Model file for the job. Use its own axes, mm. A direction names the side the tool comes from. Give positions to 0.01 mm unless a question says otherwise; leave off trailing zeros. Loops run counter-clockwise (first coordinate to the right, second up) from the corner with the lowest first, then second, coordinate; pieces in that order, holes last. Notation, with made-up numbers: (-28, 25.5) - (10, 25.5) arc R14 ccw to (10, 40.5) - close; hole circle Ø6 at (73.5, -14.75). An arc over 180 degrees is marked (long way). Answer as CSV lines item,"result". Start each with the question number.
Item 1: Saw through at B-B on z = 0. Give the cut face in (x, y) (3 decimals), plus the area to 3 significant figures.
Item 2: Drill centre lines: L1, parallel to X at y = -0.1, z = 1.5; L2, parallel to Z at x = 10.5, y = -0.2; L3, parallel to X at y = -0.9, z = 7.5. Where is each one in solid material? Low to high. Write a range as from..to.
Item 3: Saw through at D-D on z = -11.5. Give the cut face in (x, y), plus the area to 3 significant figures.
Item 4: Pin check, flat tip, straight feed: pin 1 (0.6 mm diameter, centred on y = -1, z = -7, fed in from +X). Stop position of the tip, or through.
Item 5: Pull direction Z, two halves, no side cores. Call faces 3 (the flat face through (6.747, -0.986, -3.44)), 4 (the cylindrical face through (-0.519, -0.986, -17.993)), 5 (the flat face through (0, 0, 1)): pulls with the +Z half, pulls with the -Z half, needs draft (parallel to the pull), parting line crosses it, or undercut.
Item 6: Tool access for faces 1 (the flat face through (-6.65, -0.99, -3.67)), 2 (the flat face through (0, -2, 1)): list every direction of +Z, -Z, +X, -X, +Y, -Y with a clear straight run to the whole face (end or side of a thin tool).
Item 7: Saw through at C-C on y = -0.5. State how many separate pieces and enclosed holes the cut face has, plus the area to 3 significant figures.
Item 8: Saw through at A-A on z = 16.5. Give the cut face in (x, y), plus the area to 3 significant figures.
from build123d import *

# Parameters (mm, degrees)
F1_R     = 18
F1_R_2   = 15.375
F2_DEPTH = 2
F3_DEPTH = 2


with BuildPart() as f2:
    # F0 (on Front) + F1 (on Front) → F2 (new body)
    with BuildSketch(Plane.XZ):
        Polygon((-19.759701, 18.612917), (-19.777608, 18.638063), (-19.78312, 18.635015), (-19.838238, 18.599201), (-19.84375, 18.595391), (-19.339382, 17.290085), (-14.268196, 4.150538), (-13.75283, 2.817952), (-13.962278, 2.907538), (-15.865373, 3.71508), (-16.047263, 3.792271), (-16.052775, 3.786734), (-16.102355, 3.723335), (-16.106496, 3.716452), (-15.529103, 2.9861), (-9.7441, -4.321632), (-9.165336, -5.053381), (-7.495159, -7.521448), (-7.584719, -7.543521), (-8.051876, -7.553147), (-8.541055, -7.579309), (-8.64169, -7.611034), (-8.356422, -8.069885), (-5.541086, -12.599518), (-5.259984, -13.050114), (-5.24068, -13.105257), (-5.03809, -13.466293), (-4.838268, -13.77635), (-4.819015, -13.806678), (-4.638472, -14.096086), (-2.836012, -17.000982), (-2.655468, -17.291736), (-1.86309, -17.366158), (-2.00091, -16.493846), (-3.376193, -7.774991), (-3.513988, -6.901307), (-3.62839, -6.829654), (-4.295343, -6.427292), (-4.989855, -6.00837), (-5.116652, -5.929808), (-5.2324, -5.854014), (-6.355512, -5.125034), (-6.465748, -5.053381), (-6.497472, -4.820488), (-6.808902, -2.487473), (-6.840576, -2.240788), (-6.338951, -2.426818), (-1.459332, -4.229303), (-0.975639, -4.408449), (-0.966013, -4.848047), (-0.952221, -9.157183), (-0.928802, -9.578873), (-0.796493, -9.667062), (-0.363779, -9.887534), (0.114376, -9.981235), (0.566395, -9.855835), (0.938454, -9.609176), (1.050087, -9.512706), (1.050087, -4.407078), (1.536522, -4.223791), (6.418834, -2.391004), (6.919214, -2.203577), (6.887464, -2.429612), (6.603492, -4.478757), (6.582918, -4.675784), (6.573266, -4.754347), (6.452108, -5.064404), (6.210808, -5.289017), (6.143244, -5.326228), (6.055106, -5.374462), (5.199355, -5.922924), (5.11114, -5.979439), (5.003648, -6.045581), (4.333951, -6.43829), (3.661435, -6.832422), (3.553943, -6.901307), (3.410661, -7.805293), (1.989887, -16.817696), (1.847952, -17.717541), (2.517673, -17.571466), (2.709215, -17.261408), (4.635703, -14.160856), (4.830013, -13.852169), (4.845202, -13.825957), (5.097348, -13.354685), (5.120792, -13.303707), (5.421198, -12.817246), (8.345424, -8.093304), (8.636254, -7.623404), (8.528558, -7.594498), (8.031226, -7.576566), (7.577836, -7.553147), (7.492492, -7.522845), (9.188704, -5.028565), (9.764776, -4.299585), (15.527782, 2.984729), (16.105124, 3.712337), (16.09979, 3.719195), (16.050006, 3.781222), (16.045688, 3.786734), (15.861284, 3.709568), (13.959586, 2.907538), (13.755624, 2.820746), (14.269466, 4.153306), (19.339306, 17.284751), (19.84375, 18.589549), (19.817588, 18.586755), (19.671538, 18.500141), (19.663156, 18.487695), (18.92046, 17.499635), (11.50112, 7.609383), (10.759694, 6.619977), (10.733532, 6.586906), (10.613644, 6.223102), (10.612374, 6.181776), (10.606786, 6.030189), (10.537952, 4.503318), (10.532364, 4.35036), (8.723122, 1.944319), (8.717534, 1.934642), (8.384032, 2.050415), (8.382508, 2.077974), (8.37438, 2.339797), (8.372856, 2.379777), (8.286242, 2.944749), (7.617714, 4.576343), (6.234176, 6.447739), (4.474489, 7.867193), (3.082671, 8.572551), (2.592095, 8.704885), (2.714727, 9.290609), (3.347263, 12.166651), (3.923284, 14.594637), (4.019728, 14.955825), (3.862629, 15.030247), (2.64447, 15.287803), (1.393957, 15.372972), (0, 13.366205), (-1.320852, 15.286005), (-1.918233, 15.225827), (-3.001366, 15.015007), (-3.598062, 14.824761), (-3.77444, 14.722907), (-3.6449, 14.281963), (-3.07025, 11.840007), (-2.571445, 9.225839), (-2.477694, 8.696757), (-2.965526, 8.557565), (-4.340835, 7.843571), (-6.072988, 6.428435), (-7.433132, 4.572229), (-8.089087, 2.95717), (-8.174533, 2.397658), (-8.177276, 2.365985), (-8.182788, 2.160676), (-8.182788, 2.135835), (-8.239303, 2.116557), (-8.659597, 1.974621), (-8.703691, 1.958061), (-10.526827, 4.382033), (-10.532364, 4.521251), (-10.580573, 5.899252), (-10.584713, 6.037047), (-10.587457, 6.104585), (-10.801071, 6.684823), (-10.841025, 6.737147), (-11.567262, 7.704379), (-18.822619, 17.374413), (-19.547484, 18.340121), (-19.566763, 18.366283), align=None)
    with BuildSketch(Plane.XZ):
        Circle(F1_R)
        Circle(F1_R_2, mode=Mode.SUBTRACT)
    extrude(amount=F2_DEPTH)


with BuildPart() as f3:
    # F0 (on Front) → F3 (new body)
    with BuildSketch(Plane.XZ):
        Polygon((-0.644906, 15.354097), (-1.320852, 15.286005), (0, 13.366205), (1.393957, 15.372972), (1.04455, 15.396769), (0.698678, 15.396769), (0.362407, 15.396769), align=None)
        Polygon((-1.533912, 15.595678), (-1.320852, 15.286005), (-0.644906, 15.354097), (0.362407, 15.396769), (0.698678, 15.396769), (1.04455, 15.396769), (1.393957, 15.372972), (1.555467, 15.605485), (0, 16.993944), align=None)
    extrude(amount=F3_DEPTH)


with BuildPart() as f2_1:
    add(f2.part)

    # F4: cut F3
    add(f3.part, mode=Mode.SUBTRACT)


solid = f2_1.part
Responses:
1,outline,"(-18, -2) - (-15.375, -2) - (-15.375, 0) - (-18, 0) - close; (-13.165, -2) - (13.166, -2) - (13.166, 0) - (-13.165, 0) - close; (15.375, -2) - (18, -2) - (18, 0) - (15.375, 0) - close"
1,area,"63.2 mm2"
2,L1,"-17.94..-15.3, -14.35..14.35, 15.3..17.94"
2,L2,"-14.62..-11.23, -3.37..4.31, 11.23..14.62"
2,L3,"-16.36..-11.41, -4.76..4.93, 11.42..16.36"
3,outline,"(-13.85, -2) - (-10.2, -2) - (-10.2, 0) - (-13.85, 0) - close; (-6.22, -2) - (-2.79, -2) - (-2.79, 0) - (-6.22, 0) - close; (2.83, -2) - (6.24, -2) - (6.24, 0) - (2.83, 0) - close; (10.2, -2) - (13.85, -2) - (13.85, 0) - (10.2, 0) - close"
3,area,"28.3 mm2"
4,pin 1,"x = 16.71"
5,face 3,"undercut"
5,face 4,"undercut"
5,face 5,"needs draft"
6,face 1,"+Y, -Y"
6,face 2,"+Z, -Z, +X, -X, -Y"
7,separate pieces,"1"
7,enclosed holes,"7"
7,area,"706 mm2"
8,outline,"(-19.03, -2) - (-18.17, -2) - (-18.17, 0) - (-19.03, 0) - close; (-7.19, -2) - (-0.54, -2) - (-0.54, 0) - (-7.19, 0) - close; (0.55, -2) - (7.19, -2) - (7.19, 0) - (0.55, 0) - close; (18.17, -2) - (19.04, -2) - (19.04, 0) - (18.17, 0) - close"
8,area,"30.1 mm2"
